Input: part model. Units: mm. Frame: model coordinates. A direction names the side the tool comes from. Give positions to 0.01 mm unless a question says otherwise; leave off trailing zeros. Write each loop counter-clockwise with the first axis right and the second up, starting at its lowest first coordinate (ties: lowest second). Pieces come first, ordered by that corner, then holes. Notation, with made-up numbers: (68.5, 33) - (80.5, 33) arc R27 cw to (80.5, 55) - close; hole circle Ø7 at (87, 86). An arc over 180 degrees is marked (long way). Answer as a JSON object with one key per item and string values. Group by question number.
from build123d import *

# Parameters (mm, degrees)
SKETCH2_W           = 51.4
SKETCH2_H           = 80
BOSS_EXTRUDE1_DEPTH = 4
SKETCH3_W           = 51.4
SKETCH3_H           = 4
BOSS_EXTRUDE2_DEPTH = 30
CUT_EXTRUDE1_DEPTH  = 101.997894739
FILLET1_R           = 5
FILLET2_R           = 3


with BuildPart() as part:
    # Sketch2 → Boss-Extrude1 (new body)
    with BuildSketch(Plane.XY):
        with Locations((25.725149861, -37.544031409)):
            Rectangle(SKETCH2_W, SKETCH2_H)
        with BuildLine():
            Line((10.075149861, -7.544031409), (10.075149861, -72.544031409))
            ThreePointArc((10.075149861, -72.544031409), (8.025149861, -74.594031409), (5.975149861, -72.544031409))
            Line((5.975149861, -72.544031409), (5.975149861, -7.544031409))
            ThreePointArc((5.975149861, -7.544031409), (8.025149861, -5.494031409), (10.075149861, -7.544031409))
        make_face(mode=Mode.SUBTRACT)
        with BuildLine():
            Line((41.375149861, -72.544031409), (41.375149861, -7.544031409))
            ThreePointArc((41.375149861, -7.544031409), (43.425149861, -5.494031409), (45.475149861, -7.544031409))
            Line((45.475149861, -7.544031409), (45.475149861, -72.544031409))
            ThreePointArc((45.475149861, -72.544031409), (43.425149861, -74.594031409), (41.375149861, -72.544031409))
        make_face(mode=Mode.SUBTRACT)
    extrude(amount=BOSS_EXTRUDE1_DEPTH)

    # Sketch3 → Boss-Extrude2 (add)
    with BuildSketch(Plane.XY.offset(4)):
        with Locations((25.725149861, 0.456147987)):
            Rectangle(SKETCH3_W, SKETCH3_H)
    extrude(amount=BOSS_EXTRUDE2_DEPTH)

    # Sketch4 → Cut-Extrude1 (cut, through all)
    with BuildSketch(Plane(origin=(0, 2.456147987, 0), x_dir=(1, 0, 0), z_dir=(0, 1, 0))):
        with BuildLine():
            Line((9.375149861, -8), (9.375149861, -31))
            ThreePointArc((9.375149861, -31), (8.025149861, -32.35), (6.675149861, -31))
            Line((6.675149861, -31), (6.675149861, -8))
            ThreePointArc((6.675149861, -8), (8.025149861, -6.65), (9.375149861, -8))
        make_face()
        with BuildLine():
            Line((42.075149861, -31), (42.075149861, -8))
            ThreePointArc((42.075149861, -8), (43.425149861, -6.65), (44.775149861, -8))
            Line((44.775149861, -8), (44.775149861, -31))
            ThreePointArc((44.775149861, -31), (43.425149861, -32.35), (42.075149861, -31))
        make_face()
    extrude(amount=-CUT_EXTRUDE1_DEPTH, mode=Mode.SUBTRACT)

    # Fillet1
    fillet1_edges = [part.edges().sort_by_distance(p)[0] for p in [
        (0.025149861, 0.456147987, 34),
        (51.425149861, 0.456147987, 34),
        (51.425149861, -77.544031409, 2),
        (0.025149861, -77.544031409, 2),
    ]]
    fillet(fillet1_edges, radius=FILLET1_R)

    # Fillet2
    fillet2_edges = [part.edges().sort_by_distance(p)[0] for p in [
        (25.725149861, -1.543852013, 4),
    ]]
    fillet(fillet2_edges, radius=FILLET2_R)


solid = part.part
1) Cut plane B-B on z = 3. Return the cut outline in (x, y).
2) Line query: line 1 along Y through (x, z) = (25, 11); line 2 along Z through (x, y) = (18.5, -38.5). Output: solid intervals per line, ascending. Write a range as from..to.
3) Mould query, pull axis X, two halves, no side actions, for faces 1 (the face through (25, -77.544, 2)), 2 (the face through (43.4, 0.48, 6.65)), 3 (the face through (49.922, 0.484, 32.574)). Classes: +X half, -X half, draft (parallel to the pull), parting line (faces both ways), or undercut.
4) Cut plane A-A on y = -62.5. Return the cut outline in (x, z).
5) Cut plane C-C on z = 10. Return the cut outline in (x, y), and give its area (3 significant figures).
6) Reachability of faces 4 (the face through (25, 0, 34)), 5 (the face through (8.05, 0.48, 32.35)), 6 (the face through (25, -37, 0)), 7 (the face through (43.38, -5.495, 1.972)), 8 (the face through (25, -1.544, 20)) from +Z, -Z, +X, -X, +Y, -Y: full face, straight path, thin tool, end or side. Return the list, or none.
7) Pin query (flat end, axial travel): P1, Ø5, axis at x = 30, y = -27.5, coming from the +Z side; P2, Ø13.5, axis at x = 30, z = 22.5, coming from the -Y side. Return the tip coordinate at first contact, or that it passes through.
Filled in:
{
 "1": {"outline": "(0.03, -72.54) arc R5 ccw to (5.03, -77.54) - (46.43, -77.54) arc R5 ccw to (51.43, -72.54) - (51.43, 2.46) - (0.03, 2.46) - close; hole (5.98, -72.54) arc R2.05 ccw to (10.08, -72.54) - (10.08, -7.54) arc R2.05 ccw to (5.98, -7.54) - close; hole (41.38, -72.54) arc R2.05 ccw to (45.48, -72.54) - (45.48, -7.54) arc R2.05 ccw to (41.38, -7.54) - close"},
 "2": {"line 1": "y = -1.54..2.46", "line 2": "z = 0..4"},
 "3": {"face 1": "draft", "face 2": "undercut", "face 3": "+X half"},
 "4": {"outline": "(0.03, 0) - (5.98, 0) - (5.98, 4) - (0.03, 4) - close; (10.08, 0) - (41.38, 0) - (41.38, 4) - (10.08, 4) - close; (45.48, 0) - (51.43, 0) - (51.43, 4) - (45.48, 4) - close"},
 "5": {"outline": "(0.03, -1.54) - (6.68, -1.54) - (6.68, 2.46) - (0.03, 2.46) - close; (9.38, -1.54) - (42.08, -1.54) - (42.08, 2.46) - (9.38, 2.46) - close; (44.78, -1.54) - (51.43, -1.54) - (51.43, 2.46) - (44.78, 2.46) - close", "area": "184 mm²"},
 "6": {"face 4": "+Z, +X, -X, +Y, -Y", "face 5": "+Y, -Y", "face 6": "-Z, +X, -X, +Y, -Y", "face 7": "+Z, -Z", "face 8": "+Z, +X, -X, -Y"},
 "7": {"P1": "stops at z = 4", "P2": "stops at y = -1.54"}
}
